```python
from build123d import *

# Parameters (mm, degrees)
SKETCH_1_R      = 4.05
SKETCH_1_R_2    = 1.6
SKETCH_1_R_3    = 5
EXTRUDE_1_DEPTH = 3


with BuildPart() as part:
    # ｽｹｯﾁ1 → ﾎﾞｽ - 押し出し1 (new body)
    with BuildSketch(Plane.XY):
        with BuildLine():
            Line((74, 13.65722438), (74, 98.779537634))
            Line((74, 98.779537634), (60, 98.779537634))
            ThreePointArc((60, 98.779537634), (56, 90.779537634), (52, 98.779537634))
            Line((52, 98.779537634), (38, 98.779537634))
            Line((38, 98.779537634), (0, 38))
            Line((0, 38), (0, 22))
            Line((0, 22), (38, 13.65722438))
            Line((38, 13.65722438), (74, 13.65722438))
        make_face()
        with Locations((8, 30)):
            Circle(SKETCH_1_R, mode=Mode.SUBTRACT)
        with Locations((44, 18.65722438)):
            Circle(SKETCH_1_R_2, mode=Mode.SUBTRACT)
        with Locations((68, 18.65722438)):
            Circle(SKETCH_1_R_2, mode=Mode.SUBTRACT)
        with Locations((44, 76.779537634)):
            Circle(SKETCH_1_R_2, mode=Mode.SUBTRACT)
        with Locations((56, 76.779537634)):
            Circle(SKETCH_1_R_3, mode=Mode.SUBTRACT)
        with Locations((68, 76.779537634)):
            Circle(SKETCH_1_R_2, mode=Mode.SUBTRACT)
        with Locations((44, 93.779537634)):
            Circle(SKETCH_1_R_2, mode=Mode.SUBTRACT)
        with Locations((68, 93.779537634)):
            Circle(SKETCH_1_R_2, mode=Mode.SUBTRACT)
    extrude(amount=-EXTRUDE_1_DEPTH)


solid = part.part
```
Could you check a few things on this model? Use its own coordinates, in mm. Give positions to 0.01 mm unless a question says otherwise; leave off trailing zeros. Write each loop counter-clockwise with the first axis right and the second up, starting at its lowest first coordinate (ties: lowest second). Pieces come first, ordered by that corner, then holes. Notation, with made-up numbers: (72.5, 88) -> (106.5, 88) arc R12 cw to (106.5, 109) -> close; hole circle Ø5 at (56.25, -39). An arc over 180 degrees is marked (long way). Write each question's results on one line, items separated by ' | '.
1. I want a section at B-B, the plane x = 56. Write out the boundary of the cut face in (y, z), then the cut area to 3 significant figures.
Check sheet entries:
outline: (13.66, -3) -> (71.78, -3) -> (71.78, 0) -> (13.66, 0) -> close; (81.78, -3) -> (90.78, -3) -> (90.78, 0) -> (81.78, 0) -> close | area: 201 mm²
2. I want a section at C-C, the plane y = 32.5. Write out the boundary of the cut face in (x, z), then the cut area to 3 significant figures.
Check sheet entries:
outline: (0, -3) -> (4.81, -3) -> (4.81, 0) -> (0, 0) -> close; (11.19, -3) -> (74, -3) -> (74, 0) -> (11.19, 0) -> close | area: 203 mm²
3. I need wall thicknesses on L1, parallel to Y at x = 44, z = -1.95; L2, parallel to Y at x = 44.5, z = -1.5; L3, parallel to Y at x = 22.5, z = -2.65. Which ranges of each line are inside material? Lowest first, please.
Check sheet entries:
L1: y = 13.66 to 17.06, 20.26 to 75.18, 78.38 to 92.18, 95.38 to 98.78 | L2: y = 13.66 to 17.14, 20.18 to 75.26, 78.3 to 92.26, 95.3 to 98.78 | L3: y = 17.06 to 73.99
4. If we mould it in two halves opening along Y, with no side actions, what happens to faces 1 (the cylindrical face through (44.9, 78.1, -1.5)), 2 (the flat face through (0, 30, -1)), 3 (the flat face through (67, 98.78, -1))? For each: released by +Y, released by -Y, zero draft, split by the parting line, or undercut.
Check sheet entries:
face 1: undercut | face 2: zero draft | face 3: released by +Y
5. I want a section at A-A, the plane x = 44. Write out the boundary of the cut face in (y, z).
Check sheet entries:
outline: (13.66, -3) -> (17.06, -3) -> (17.06, 0) -> (13.66, 0) -> close; (20.26, -3) -> (75.18, -3) -> (75.18, 0) -> (20.26, 0) -> close; (78.38, -3) -> (92.18, -3) -> (92.18, 0) -> (78.38, 0) -> close; (95.38, -3) -> (98.78, -3) -> (98.78, 0) -> (95.38, 0) -> close
6. I want a section at D-D, the plane z = -1.75. Count the separate pieces of the cut face and the enclosed holes in it, then the cut area to 3 significant figures.
Check sheet entries:
separate pieces: 1 | enclosed holes: 8 | area: 4,740 mm²
